```python
from build123d import *

# Parameters (mm, degrees)
F0_R      = 115
F1_DEPTH  = 2
F2_R      = 107
F2_R_2    = 105
F3_DEPTH  = 15
F5_R      = 110
F6_DEPTH  = 1.5
F7_R      = 1
F6_FACE_R = 105
F9_DEPTH  = 12
F11_DEPTH = 15
F13_DEPTH = 15


with BuildPart() as f1:
    # F0 (on Front) → F1 (new body)
    with BuildSketch(Plane.XZ):
        Circle(F0_R)
    extrude(amount=F1_DEPTH)

    # F2 (on face) → F3 (join)
    with BuildSketch(Plane.XZ.offset(2)):
        Circle(F2_R)
        Circle(F2_R_2, mode=Mode.SUBTRACT)
    extrude(amount=F3_DEPTH)

    # F5 (on offset) → F6 (join)
    with BuildSketch(Plane.XZ.offset(13)):
        Circle(F5_R)
    extrude(amount=F6_DEPTH)

    # F7
    f7_edges = [f1.edges().sort_by_distance(p)[0] for p in [
        (-115, 0, 0),
    ]]
    fillet(f7_edges, radius=F7_R)

    # F6_face (on face) → F9 (cut)
    with BuildSketch(Plane.XZ.offset(14.5)):
        Circle(F6_FACE_R)
    extrude(amount=-F9_DEPTH, mode=Mode.SUBTRACT)

    # F10 (on face) → F11 (cut)
    with BuildSketch(Plane(origin=(0, 0, 0), x_dir=(-1, 0, 0), z_dir=(0, 1, 0))):
        Polygon((-17.259745, 100.488558), (-38.544491, 80.841102), (41.955505, 81.113979), align=None)
        Polygon((83.706349, 59.829235), (39.226692, 72.927542), (97.623304, 0), align=None)
        Polygon((102.808043, -13.302966), (68.425, 21.352965), (58.601268, -79.613134), align=None)
        Polygon((25.309743, -97.623304), (54.235172, -49.323305), (-53.825844, -84.524997), align=None)
        Polygon((-81.386864, -48.231781), (-54.37161, -76.611444), (6.208051, -55.326693), align=None)
        Polygon((-102.671608, 0), (-88.481776, -46.321612), (-86.844489, 45.366522), align=None)
        Polygon((-33.905506, 75.383477), (-72.654657, 67.197032), (-80.568217, 24.900423), align=None)
    extrude(amount=-F11_DEPTH, mode=Mode.SUBTRACT)

    # F12 (on face) → F13 (cut)
    with BuildSketch(Plane(origin=(0, 0, 0), x_dir=(-1, 0, 0), z_dir=(0, 1, 0))):
        Polygon((16.031779, 73.473305), (-32.813981, 58.73771), (51.23347, 38.544491), align=None)
        Polygon((57.782628, 29.539406), (31.040253, 38.27161), (56.963984, -21.216525), align=None)
        Polygon((12.484324, -52.052118), (55.326689, -29.130084), (-29.539406, -25.582626), align=None)
        Polygon((-76.474994, -33.769067), (-16.713982, -47.140256), (-82.205504, 15.622457), align=None)
        Polygon((-51.369913, -6.208051), (-45.366526, 51.915679), (-70.744492, 27.629238), align=None)
        Polygon((11.665677, 33.359747), (-28.720763, 52.18856), (-41.546185, 11.529238), align=None)
        Polygon((42.22839, -10.847033), (16.577544, 29.812288), (-13.166525, 14.530932), align=None)
        Polygon((-19.169914, -21.489406), (29.402964, -12.484322), (-40.181778, 4.161441), align=None)
    extrude(amount=-F13_DEPTH, mode=Mode.SUBTRACT)


solid = f1.part
```
Read the model definition and answer for the solid it produces. Units are mm, in the model's axes. A direction names the side the tool comes from. Give positions to 0.01 mm unless a question says otherwise; leave off trailing zeros. Order: outer loops, then holes, each group sorted by start corner. A loop starts at its lowest first (then second) coordinate and runs counter-clockwise, first axis right, second up.
(1) For a pull along X with two mould halves and no side action, classify faces 1 (the flat face through (24, -13, -105)), 2 (the flat face through (48.41, -0.99, 22.45)), 3 (the cylindrical face through (-23.196, -15.732, -104.456)) as released by +X, released by -X, zero draft, split by the parting line, or undercut.
(2) Straight lines are drawn through the part: L1, parallel to Z at x = 0, y = -9; L2, parallel to Z at x = -81, y = -1.5; L3, parallel to Z at x = 43, y = -1.5. For each, find the intervals that lie inside material, in ascending order.
(3) Find section A-A (y = -6). Give the vertices of the cut face in (x, z).
(4) For faces 4 (the flat face through (-90.76, -0.99, 29.5)), 5 (the cylindrical face through (-23.846, -13.74, -107.384)), determine the directions among +Z, -Z, +X, -X, +Y, -Y from which every point of the face is accessible in a straight line to the end or side of a thin tool.
(5) Given pin 1 (5 mm diameter, centred on y = -3, z = 21, fed in from +X); pin 2 (2 mm diameter, centred on x = -27.5, z = 31, fed in from -Y); pin 3 (1 mm diameter, centred on x = -4, y = -14.5, fed in from -Z), each flat-ended and moving along its own axis, determine where each tip first touches the part or whether it passes through.
(6) Find section B-B (z = -17). Give the number of separate pieces and of enclosed holes in the cut face, plus the area to 3 significant figures.
Result sheet:
1. face 1: zero draft
1. face 2: undercut
1. face 3: split by the parting line
2. L1: z = -107 to -105, 105 to 107
2. L2: z = -81.63 to -46.02, 8.68 to 20.76, 60.63 to 81.63
2. L3: z = -106.66 to -86.32, -81 to -72.62, -51.34 to -41.26, -21.95 to 65.54, 73.46 to 106.66
3. outline: circle Ø214 at (0, 0); hole circle Ø210 at (0, 0)
4. face 4: +Y, -Y
4. face 5: -Y
5. pin 1: stops at x = 113.47
5. pin 2: stops at y = -2
5. pin 3: stops at z = -109.94
6. separate pieces: 6
6. enclosed holes: 0
6. area: 314 mm2
